from build123d import *

# Parameters (mm, degrees)
SKETCH1_W                = 65
SKETCH1_H                = 55
BOSS_EXTRUDE1_DEPTH      = 4
SKETCH2_W                = 2.5
SKETCH2_H                = 55
BOSS_EXTRUDE2_DEPTH      = 60
SKETCH2_3_W              = 2.5
SKETCH2_3_H              = 55
BOSS_EXTRUDE3_DEPTH      = 30
BOSS_EXTRUDE4_DEPTH      = 2.5
BOSS_EXTRUDE4_DEPTH_BACK = 2.5
SKETCH4_R                = 10
BOSS_EXTRUDE5_START      = -62.5
SKETCH4_2_R              = 10
BOSS_EXTRUDE5_DEPTH      = 5
CUT_EXTRUDE1_DEPTH       = 113.403083271
CUT_EXTRUDE1_DEPTH_BACK  = 113.403083271
SKETCH5_R                = 3


with BuildPart() as part:
    # Sketch1 → Boss-Extrude1 (new body)
    with BuildSketch(Plane(origin=(0, 0, 0), x_dir=(1, 0, 0), z_dir=(0, 1, 0))):
        Rectangle(SKETCH1_W, SKETCH1_H)
    extrude(amount=BOSS_EXTRUDE1_DEPTH)

    # Sketch2 → Boss-Extrude2 (add)
    with BuildSketch(Plane(origin=(0, 4, 0), x_dir=(1, 0, 0), z_dir=(0, 1, 0))):
        with Locations((-28.75, 0)):
            Rectangle(SKETCH2_W, SKETCH2_H)
        with Locations((28.75, 0)):
            Rectangle(SKETCH2_W, SKETCH2_H)
    extrude(amount=BOSS_EXTRUDE2_DEPTH)

    # Sketch2_3 → Boss-Extrude3 (add)
    with BuildSketch(Plane(origin=(0, 4, 0), x_dir=(1, 0, 0), z_dir=(0, 1, 0))):
        with Locations((-31.25, 0)):
            Rectangle(SKETCH2_3_W, SKETCH2_3_H)
        with Locations((31.25, 0)):
            Rectangle(SKETCH2_3_W, SKETCH2_3_H)
    extrude(amount=BOSS_EXTRUDE3_DEPTH)

    # Sketch4 → Boss-Extrude4 (add, two sides: drawn at the far end of the back side and taken through both)
    with BuildSketch(Plane.ZY.offset(30).offset(-BOSS_EXTRUDE4_DEPTH_BACK)):
        with BuildLine():
            Line((23.388987302, 56.500283138), (-23.388987302, 56.500283138))
            ThreePointArc((-23.388987302, 56.500283138), (0, 103.527582425), (23.388987302, 56.500283138))
        make_face()
        with Locations((0, 74.19768631)):
            Circle(SKETCH4_R, mode=Mode.SUBTRACT)
    extrude(amount=BOSS_EXTRUDE4_DEPTH + BOSS_EXTRUDE4_DEPTH_BACK)

    # Sketch4_2 → Boss-Extrude5 (add)
    with BuildSketch(Plane.ZY.offset(30).offset(BOSS_EXTRUDE5_START)):
        with BuildLine():
            Line((23.388987302, 56.500283138), (-23.388987302, 56.500283138))
            ThreePointArc((-23.388987302, 56.500283138), (0, 103.527582425), (23.388987302, 56.500283138))
        make_face()
        with Locations((0, 74.19768631)):
            Circle(SKETCH4_2_R, mode=Mode.SUBTRACT)
    extrude(amount=BOSS_EXTRUDE5_DEPTH)

    # Sketch5 → Cut-Extrude1 (cut, two sides: drawn at the far end of the back side and taken through both)
    with BuildSketch(Plane.XZ.offset(-CUT_EXTRUDE1_DEPTH_BACK)):
        with Locations(Location((0, 10, 0), (0, 0, 270))):
            Circle(SKETCH5_R)
        with Locations(Location((0, -10, 0), (0, 0, 270))):
            Circle(SKETCH5_R)
    extrude(amount=CUT_EXTRUDE1_DEPTH + CUT_EXTRUDE1_DEPTH_BACK, mode=Mode.SUBTRACT)


solid = part.part
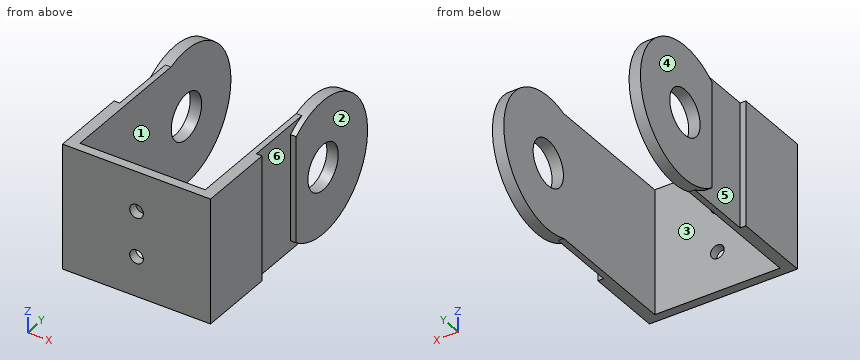
The listing builds one solid part. Answer for the finished solid, in the listing's coordinates (mm). Face numbers are marked on the shaded views. A direction names the side the tool comes from. Coordinates: 2 decimals unless noted, no trailing zeros. Write each loop counter-clockwise with the first axis right and the second up, starting at its lowest first coordinate (ties: lowest second). Pieces come first, ordered by that corner, then holes. Notation, with made-up numbers: M -23.5,-4.75 L -5.5,-4.75 A37 ccw -5.5,32.25 Z; hole C 50.25,57.5 d3. An arc over 180 degrees is marked long. Put each result on its own line as item: value. Start each with the question number.
1. A cutting plane is placed at A-A on x = 0. Write down the section's boundary in (y, z).
2. A cutting plane is placed at C-C on y = 80. Write down the section's boundary in (x, z).
3. Consider line 1 (Z direction, x = 0, y = 2); line 2 (Y direction, x = -31, z = 0); line 3 (X direction, y = 36, z = -12). Determine where each line is inside the solid, lowest interval first. Write a range as from..to.
4. Which of the six approach directions +Z, -Z, +X, -X, +Y, -Y give full straight-line access (tool end or side, diameter ignored) to the marked faces 1 and 2?
5. A cutting plane is placed at D-D on z = -1.5. Write down the section's boundary in (x, y), then the cut area to 3 significant figures.
6. Flat-ended cylindrical pins translate along their axes: P1, Ø8, axis at x = 24, y = 61, coming from the +Z side; P2, Ø4, axis at y = 52, z = 16.5, coming from the -X side; P3, Ø3, axis at x = 25, z = 19, coming from the +Y side. Find the tip coordinate at first contact, or state that the pin passes through.
7. A cutting plane is placed at B-B on y = 14.5. Write down the section's boundary in (x, z).
8. For a pull along Y with two mould halves and no side action, classify the marked faces 3, 4, 5 and 6 as pulls with the +Y half, pulls with the -Y half, needs draft (parallel to the pull), parting line crosses it, or undercut.
Resolved:
1. outline: M 0,-27.5 L 4,-27.5 L 4,-13 L 0,-13 Z; M 0,-7 L 4,-7 L 4,7 L 0,7 Z; M 0,13 L 4,13 L 4,27.5 L 0,27.5 Z
2. outline: M -32.5,-28.75 L -27.5,-28.75 L -27.5,-8.14 L -32.5,-8.14 Z; M -32.5,8.14 L -27.5,8.14 L -27.5,28.75 L -32.5,28.75 Z; M 27.5,-28.75 L 32.5,-28.75 L 32.5,-8.14 L 27.5,-8.14 Z; M 27.5,8.14 L 32.5,8.14 L 32.5,28.75 L 27.5,28.75 Z
3. line 1: z = -27.5..-13, -7..7, 13..27.5
3. line 2: y = 0..34, 56.5..64.2, 84.2..103.53
3. line 3: x = -30..-27.5, 27.5..30
4. face 1: +Z, -Z, +Y
4. face 2: +Z, -Z, +X, +Y, -Y
5. outline: M -32.5,0 L 32.5,0 L 32.5,34 L 30,34 L 30,56.5 L 32.5,56.5 L 32.5,64.31 L 27.5,64.31 L 27.5,4 L -27.5,4 L -27.5,64.31 L -32.5,64.31 L -32.5,56.5 L -30,56.5 L -30,34 L -32.5,34 Z; M -32.5,84.08 L -27.5,84.08 L -27.5,103.49 L -32.5,103.49 Z; M 27.5,84.08 L 32.5,84.08 L 32.5,103.49 L 27.5,103.49 Z
5. area: 945 mm2
6. P1: stops at z = 27.5
6. P2: stops at x = -30
6. P3: stops at y = 4
7. outline: M -32.5,-27.5 L -27.5,-27.5 L -27.5,27.5 L -32.5,27.5 Z; M 27.5,-27.5 L 32.5,-27.5 L 32.5,27.5 L 27.5,27.5 Z
8. face 3: pulls with the +Y half
8. face 4: needs draft
8. face 5: undercut
8. face 6: undercut
